Source: CAD feature listing. Evaluate the final solid. Frame: model axes, mm. A direction names the side the tool comes from. Round coordinates to 2 decimals unless told otherwise and drop trailing zeros. Write each loop counter-clockwise with the first axis right and the second up, starting at its lowest first coordinate (ties: lowest second). Pieces come first, ordered by that corner, then holes. Notation, with made-up numbers: M 88.5,-12 L 133.5,-12 A22 ccw 133.5,12 Z; hole C 86,64.5 d8. An arc over 180 degrees is marked long. Use a Markdown table: item, result.
Autodesk Inventor part; units mm, degrees
ref_plane "YZ Plane" through (0, 0, 0) normal (1, 0, 0) x (0, 1, 0)
ref_plane "XZ Plane" through (0, 0, 0) normal (0, 1, 0) x (-1, 0, 0)
ref_plane "XY Plane" through (0, 0, 0) normal (0, 0, 1) x (1, 0, 0)
sketch "スケッチ1" plane through (0, 0, 0) normal (0, 0, 1) x (1, 0, 0)
  line L0 (-20, -20) -> (20, -20)
  line L1 (20, -20) -> (20, 20)
  line L2 (20, 20) -> (-20, 20)
  line L3 (-20, 20) -> (-20, -20)
  line L4 (-20, -20) -> (20, 20) construction
  line L5 (20, -20) -> (-20, 20) construction
  point P0 (0, 0)
  dimension "d0" = 40
  dimension "d1" = 40
extrude "押し出し1" add sketch "スケッチ1" along normal blind 110
sketch "スケッチ2" plane through (0, 0, 110) normal (0, 0, 1) x (1, 0, 0)
  circle A0 centre (0, 0) radius 10
  dimension "d4" = 20
extrude "押し出し2" add sketch "スケッチ2" along normal blind 8
sketch "スケッチ3" plane through (-20, -20, 0) normal (-1, 0, 0) x (0, 0, 1)
  line L0 (0, 40) -> (0, 0)
  line L1 (0, 0) -> (110, 0)
  line L2 (110, 40) -> (110, 0)
  line L3 (0, 40) -> (110, 40)
  line L4 (64, 10) -> (104, 10)
  line L5 (104, 10) -> (104, 30)
  line L6 (104, 30) -> (64, 30)
  line L7 (64, 30) -> (64, 10)
  line L8 (64, 10) -> (104, 30) construction
  line L9 (104, 10) -> (64, 30) construction
  point P0 (0, 20)
  point P1 (84, 20)
  point P2 (0, 20)
  point P3 (84, 20)
  dimension "d7" = 20
  dimension "d8" = 40
  dimension "d9" = 6
hole "穴1" at (-20, 10, 64) at (-20, -10, 64) at (-20, -10, 104) at (-20, 10, 104) direction (1, 0, 0) diameter 3.3 depth 8.8
properties part number "Diode_Laser"
Q1. Section C-C on z = 64. Return loops of the section in (x, y).
Results are:
| item | result |
|---|---|
| outline | M -20,-20 L 20,-20 L 20,20 L -20,20 L -20,11.65 L -11.2,11.65 L -11.2,8.35 L -20,8.35 L -20,-8.35 L -11.2,-8.35 L -11.2,-11.65 L -20,-11.65 Z |
Q2. Reachability of faces 4 (the flat face through (0, 0, 0)), 5 (the cylindrical face through (-15.54, 9.93, 62.35)), 6 (the cylindrical face through (-2.17, 9.76, 113.94)) from +Z, -Z, +X, -X, +Y, -Y: full face, straight path, thin tool, end or side. Return the list, or none.
Results are:
| item | result |
|---|---|
| face 4 | -Z, +X, -X, +Y, -Y |
| face 5 | -X |
| face 6 | +Z |
Q3. Section D-D on x = 16.5. Return loops of the section in (y, z), plus the area to 3 significant figures.
Results are:
| item | result |
|---|---|
| outline | M -20,0 L 20,0 L 20,110 L -20,110 Z |
| area | 4,400 mm^2 |
Q4. First-contact query: pin 1 Ø2.5 at (y, z) = (10, 104) entering from -X; pin 2 Ø1 at (x, y) = (11.5, -4.5) entering from +Z. Flat tips, straight axial feed; report the tip coordinate or a pass-through.
Results are:
| item | result |
|---|---|
| pin 1 | x = -11.2 |
| pin 2 | z = 110 |
Q5. Mould query, pull axis Y, two halves, no side actions, for faces 1 (the flat face through (0, 20, 54)), 2 (the flat face through (-11.2, 10, 64)), 3 (the flat face through (-20, 0, 54)). Classes: +Y half, -Y half, draft (parallel to the pull), parting line (faces both ways), or undercut.
Results are:
| item | result |
|---|---|
| face 1 | +Y half |
| face 2 | undercut |
| face 3 | draft |
Q6. Section A-A on y = 0. Return loops of the section in (x, z).
Results are:
| item | result |
|---|---|
| outline | M -20,0 L 20,0 L 20,110 L 10,110 L 10,118 L -10,118 L -10,110 L -20,110 Z |
Q7. Line query: L1, parallel to Y at x = -17.5, z = 64; L2, parallel to Z at x = -14.75, y = 10; L3, parallel to Z at x = -12, y = -2. Output: solid intervals per line, ascending.
Results are:
| item | result |
|---|---|
| L1 | -20 to -11.65, -8.35 to 8.35, 11.65 to 20 |
| L2 | 0 to 62.35, 65.65 to 102.35, 105.65 to 110 |
| L3 | 0 to 110 |
